Source: CAD feature listing. Evaluate the final solid. Frame: model axes, mm. Face numbers are marked on the shaded views. Round coordinates to 2 decimals unless told otherwise and drop trailing zeros. Loops run counter-clockwise (first coordinate to the right, second up) from the corner with the lowest first, then second, coordinate; pieces in that order, holes last. Notation, with made-up numbers: (62, 53.25) -> (110, 53.25) arc R12 ccw to (110, 63.25) -> close; hole circle Ø1 at (-26, -38). An arc over 180 degrees is marked (long way). Write item = value, one per line.
from build123d import *

# Parameters (mm, degrees)
F0_W     = 150.700152
F0_H     = 74.61378
F1_DEPTH = 12.7
F3_D     = 6.35
F5_D     = 12.7


with BuildPart() as f1:
    # F0 (on Top) → F1 (new body)
    with BuildSketch(Plane.XY):
        Rectangle(F0_W, F0_H)
    extrude(amount=F1_DEPTH)

    # F3 (through all)
    with Locations(Plane.XY.offset(12.7)):
        with Locations((75.350076, 0)):
            Hole(F3_D / 2)

    # F5 (through all)
    with Locations(Plane.XY.offset(12.7)):
        with Locations((-75.350076, 0)):
            Hole(F5_D / 2)


solid = f1.part
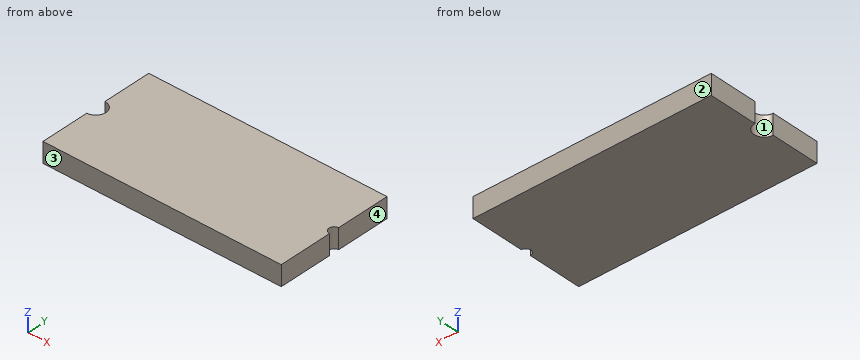
1. Mould query, pull axis Y, two halves, no side actions, for the marked faces 1, 2, 3 and 4. Classes: released by +Y, released by -Y, zero draft, split by the parting line, or undercut.
Evaluation:
face_1 = undercut
face_2 = released by +Y
face_3 = released by -Y
face_4 = zero draft
2. Line query: probe 1 along X at (y, z) = (4.5, 5). Output: solid intervals per line, ascending. Write a range as from..to.
Evaluation:
probe_1 = -70.87..75.35
3. Section query A-A (y = 0). Return the cut outline in (x, z), then the cut area to 3 significant figures.
Evaluation:
outline = (-69, 0) -> (72.18, 0) -> (72.18, 12.7) -> (-69, 12.7) -> close
area = 1,790 mm²
4. Contact query for a flat-ended pin moving along its axis: pin 1 Ø2 at (x, y) = (5, 12.5) entering from -Z. Output: stop coordinate, or through.
Evaluation:
pin_1 = 0
